Here's how the part is built. I have some questions about the finished solid (model axes, mm). A direction names the side the tool comes from. Round coordinates to 2 decimals unless told otherwise and drop trailing zeros. Loops run counter-clockwise (first coordinate to the right, second up) from the corner with the lowest first, then second, coordinate; pieces in that order, holes last. Notation, with made-up numbers: M 87,-27 L 101,-27 A20 cw 101,10 Z; hole C -34,20.5 d10. An arc over 180 degrees is marked long. Answer as a JSON object with one key per item and string values.
Autodesk Inventor part; units mm, degrees
ref_plane "YZ Plane" through (0, 0, 0) normal (1, 0, 0) x (0, 1, 0)
ref_plane "XZ Plane" through (0, 0, 0) normal (0, 1, 0) x (-1, 0, 0)
ref_plane "XY Plane" through (0, 0, 0) normal (0, 0, 1) x (1, 0, 0)
sketch "Sketch1" plane through (0, 0, 0) normal (0, 0, 1) x (1, 0, 0)
  line L0 (0, 0) -> (0, 23.7553)
  line L1 (0, 0) -> (15.875, 0)
  line L2 (0, 23.7553) -> (7.9451, 23.7553)
  line L3 (7.9451, 23.7553) -> (15.875, 0)
  line L4 (7.9451, 23.7553) -> (31.7005, 23.7553) construction
  line L5 (0, 23.7553) -> (0, 15.8369)
  line L6 (0, 0) -> (0, 7.9184)
  dimension "d0" = 23.7553
  dimension "d1" = 15.875
  dimension "d2" = 7.9451
  dimension "d10" = 7.9185
extrude "Extrusion2" add sketch "Sketch1" along normal blind 3.236
sketch "Sketch3" plane through (0, 0, 3.236) normal (0, 0, 1) x (1, 0, 0)
  line L0 (15.875, 0) -> (7.9451, 23.7553)
  line L1 (0, 0) -> (15.875, 0)
  line L2 (7.9451, 23.7553) -> (7.9451, 0)
  line L3 (7.9451, 23.7553) -> (0, 23.7553)
  line L4 (0, 23.7553) -> (0, 15.8369)
  line L5 (0, 23.7553) -> (0, 0)
  line L6 (0, 15.8369) -> (0, 7.9184)
  circle A0 centre (3.9726, 19.7961) radius 2.4879
  dimension "d17" = 4.9759
extrude "Extrusion3" add sketch "Sketch3" along normal blind 1.7577 contours A0
pattern_linear "Rectangular Pattern2" count 3 spacing 7.7978 along (0, -1, 0) of "Extrusion3"
shell "Shell1" thickness 1.4732 removed faces 1 at (7.94, 7.9185, 0)
sketch "Sketch5" plane through (13.8301, 1.4732, 1.7628) normal (0, 0, -1) x (-1, 0, 0)
  circle A0 centre (5.9587, 6.6262) radius 2.4498
  circle A1 centre (5.9587, 6.6262) radius 3.0259
  circle A2 centre (9.8576, 2.7273) radius 2.4879 construction
  circle A3 centre (9.8576, 10.5251) radius 2.4879 construction
  line L0 (9.8576, 10.5251) -> (2.0598, 10.5251) construction
  line L1 (2.0598, 10.5251) -> (2.0598, 2.7273) construction
  line L2 (2.0598, 2.7273) -> (9.8576, 2.7273) construction
  line L3 (9.8576, 2.7273) -> (9.8576, 10.5251) construction
  line L4 (9.8576, 10.5251) -> (2.0598, 2.7273) construction
  point P0 (13.8301, -1.4732)
  dimension "d39" = 7.7978
  dimension "d40" = 7.7978
  dimension "d41" = 4.8997
extrude "Extrusion4" add sketch "Sketch5" along normal up to surface (1.7628 mm away)
pattern_linear "Rectangular Pattern3" count 2 spacing 7.7978 along (0, 1, 0) of "Extrusion4"
sketch "Sketch6" plane through (0, 0, 0) normal (0, 0, -1) x (-1, 0, 0)
  circle A0 centre (-3.9726, 4.2005) radius 2.4879
  line L0 (-3.9726, 4.2005) -> (-11.7704, 4.2005) construction
  arc A1 (-12.5581, 1.8406) -> (-10.9826, 6.5604) centre (-11.7704, 4.2005) ccw
  circle A2 centre (-7.8715, 8.0994) radius 3.0259
  line L1 (-10.9826, 6.5604) -> (-20.4448, 9.7191)
  line L2 (-12.5581, 1.8406) -> (-25.2023, 6.0614)
  line L3 (-25.2023, 6.0614) -> (-20.4448, 9.7191)
  line L4 (-15.875, 0) -> (-10.8097, 15.174)
  point P0 (0, 0)
  dimension "d42" = 7.7978
extrude "Extrusion5" cut sketch "Sketch6" against normal up to surface (1.7628 mm away) contours A1 L2 L4 L1 | L2 L3 L1 L4
sketch "Sketch7" plane through (0, 0, 0) normal (0, 0, -1) x (-1, 0, 0)
  circle A0 centre (-3.9726, 11.9983) radius 2.4879
  line L0 (-3.9726, 11.9983) -> (-11.7704, 11.9983) construction
  circle A1 centre (-11.7704, 11.9983) radius 2.4879
  circle A2 centre (-7.8715, 8.0994) radius 3.0259
  line L1 (-13.4141, 7.3721) -> (-10.8097, 15.174)
  line L2 (-11.0726, 14.3864) -> (-8.7367, 21.384)
  line L3 (-8.7367, 21.384) -> (-11.249, 21.384)
  line L4 (-11.249, 21.384) -> (-14.0474, 13.0007)
  line L5 (-25.9039, 14.0934) -> (-10.7493, 9.0346)
  line L6 (-24.9299, 19.014) -> (-10.9826, 14.3582)
  line L7 (-24.9299, 19.014) -> (-25.9039, 14.0934)
  line L8 (-10.7493, 9.0346) -> (-11.1181, 9.5974)
  line L9 (-12.0167, 6.9056) -> (-9.7949, 13.5613)
  point P0 (0, 0)
  dimension "d45" = 7.7978
extrude "Extrusion6" cut sketch "Sketch7" against normal up to surface (1.7628 mm away) contours L1 A1 L9 | A1 L9 | L5 L9 L8 | L5 L7 L6 L4 A1 | A1 L1 | L9 L5 A1 | L4 L6 A1 | L6 L4 L3 L2 L1
properties part number "3x1 diagonal" material "ABS Plastic"
Item 1: If I drill on L1, parallel to Y at x = 1.75, z = 1.55; L2, parallel to Z at x = 9.25, y = 2; L3, parallel to Z at x = 3.5, y = 21.75, over which ranges is the centre line in solid material (lowest first)? Write a range as from..to.
Solution:
{"L1": "y = 0..1.47, 22.28..23.76", "L2": "z = 1.76..3.24", "L3": "z = 1.76..4.99"}
Item 2: We'd pull the mould along Y, two halves only. Please class faces 6 (the face through (4, 12, 3.52)), 7 (the face through (12.706, 7.136, 0.869)), 8 (the face through (5, 8, 0)), 9 (the face through (11.94, 9.43, 0.87)): +Y half, -Y half, draft (parallel to the pull), parting line (faces both ways), or undercut.
Solution:
{"face 6": "undercut", "face 7": "undercut", "face 8": "draft", "face 9": "+Y half"}
Item 3: I want a section at D-D on x = 7.25. List the corners of the cut face in (y, z) for me, plus the area to 3 significant figures.
Solution:
{"outline": "M 0,0 L 1.47,0 L 1.47,1.76 L 5.14,1.76 L 5.14,0 L 5.73,0 L 5.73,1.76 L 10.47,1.76 L 10.47,0 L 11.06,0 L 11.06,1.76 L 12.94,1.76 L 12.94,0 L 13.53,0 L 13.53,1.76 L 18.27,1.76 L 18.27,0 L 18.86,0 L 18.86,1.76 L 21.18,1.76 L 21.18,0 L 23.76,0 L 23.76,3.24 L 0,3.24 Z", "area": "46.3 mm2"}
Item 4: I want a section at B-B on z = 2. List the corners of the cut face in (x, y) for me (1 decimal).
Solution:
{"outline": "M 0,0 L 15.9,0 L 7.9,23.8 L 0,23.8 Z; hole C 4,4.2 d2; hole C 4,12 d2; hole C 4,19.8 d2"}
Item 5: For faces 1 (the face through (4, 12, 4.994)), 2 (the face through (14.281, 2.416, 0.869)), 3 (the face through (6, 14, 0)), 4 (the face through (7.44, 20.62, 0.87)), 5 (the face through (3.43, 6.63, 4.1)), which set-ups out of +Z, -Z, +X, -X, +Y, -Y let a thin tool reach every point of the face, with its end or its side?
Solution:
{"face 1": "+Z, +X, -X, +Y, -Y", "face 2": "-Z, +Y", "face 3": "-Z, +X, -X, +Y, -Y", "face 4": "-Z", "face 5": "+Z"}
Item 6: I want a section at A-A on z = 0.4. Count the separate pieces of the cut face and the enclosed holes in it, plus the area to 3 significant figures.
Solution:
{"separate pieces": "3", "enclosed holes": "2", "area": "99.8 mm2"}
Item 7: For P1, Ø1.4, axis at y = 12, z = 1, coming from the +X side; P2, Ø4.5, axis at x = 7.87, y = 8.1, coming from the +Z side; P3, Ø0.6, axis at x = 4.5, y = 19.5, coming from the -Z side; P4, Ø2, axis at x = 12.5, y = 19, coming from the -Z side, each with a flat end and sliding along its axis, tell me the tip position at first contact or that it passes through.
Solution:
{"P1": "stops at x = 1.47", "P2": "stops at z = 3.24", "P3": "stops at z = 3.52", "P4": "passes through"}
